```python
from build123d import *

# Parameters (mm, degrees)
F0_R          = 20
F0_R_2        = 17.5
F1_DEPTH      = 135
F2_R          = 30
F2_R_2        = 26.9985
F2_R_3        = 17.5
F3_DEPTH      = 25
F4_R          = 26.9965
F4_R_2        = 24
F4_R_3        = 17.5
F5_DEPTH      = 12
F6_R          = 25.5
F6_R_2        = 22.4965
F6_R_3        = 20
F6_R_4        = 17.5
F7_DEPTH      = 25
F8_R          = 21.9965
F8_R_2        = 17.5
F9_DEPTH      = 12
F10_S5_R      = 20
F10_T6_DEPTH  = 38
F10_S11_R     = 20
F10_T12_DEPTH = 44


# Not quite as in the source:
# - a fillet or chamfer that OpenCascade refuses, or shapes differently, is made with other operations: its cross-section is extruded or revolved along the edge and cut away or added


with BuildPart() as f1:
    # F0 (on Top) → F1 (new body)
    with BuildSketch(Plane.XY):
        Circle(F0_R)
        Circle(F0_R_2, mode=Mode.SUBTRACT)
    extrude(amount=F1_DEPTH)

    # F2 (on Top) → F3 (join)
    with BuildSketch(Plane.XY):
        Circle(F2_R)
        Circle(F2_R_2, mode=Mode.SUBTRACT)
        Circle(F2_R_2)
        Circle(F2_R_3, mode=Mode.SUBTRACT)
    extrude(amount=-F3_DEPTH)

    # F4 (on face) → F5 (cut)
    with BuildSketch(Plane(origin=(0, 0, -25), x_dir=(1, 0, 0), z_dir=(0, 0, -1))):
        Circle(F4_R)
        Circle(F4_R_2, mode=Mode.SUBTRACT)
        Circle(F4_R_2)
        Circle(F4_R_3, mode=Mode.SUBTRACT)
    extrude(amount=-F5_DEPTH, mode=Mode.SUBTRACT)

    # F6 (on face) → F7 (join)
    with BuildSketch(Plane.XY.offset(135)):
        Circle(F6_R)
        Circle(F6_R_2, mode=Mode.SUBTRACT)
        Circle(F6_R_2)
        Circle(F6_R_3, mode=Mode.SUBTRACT)
        Circle(F6_R_3)
        Circle(F6_R_4, mode=Mode.SUBTRACT)
    extrude(amount=F7_DEPTH)

    # F8 (on face) → F9 (cut)
    with BuildSketch(Plane.XY.offset(160)):
        Circle(F8_R)
        Circle(F8_R_2, mode=Mode.SUBTRACT)
    extrude(amount=-F9_DEPTH, mode=Mode.SUBTRACT)

    # F10: chamfer of 10 on 2 edges, made by hand


with BuildPart() as f10_tool2:
    # F10_s3 → F10_t4 (revolve)
    with BuildSketch(Plane.XZ):
        Polygon((15.5, 135), (25.5, 145), (25.5, 135), align=None)
    revolve(axis=Axis((0, 0, 135), (0, 0, 1)))

    # F10_s5 → F10_t6 (cut, symmetric)
    with BuildSketch(Plane.XY.offset(140)):
        Circle(F10_S5_R)
    extrude(amount=F10_T6_DEPTH, both=True, mode=Mode.SUBTRACT)


with BuildPart() as f1_1:
    add(f1.part)

    # F10_t1: cut F10_tool2
    add(f10_tool2.part, mode=Mode.SUBTRACT)


with BuildPart() as f10_tool8:
    # F10_s9 → F10_t10 (revolve)
    with BuildSketch(Plane.XZ):
        Polygon((20, 0), (30, -10), (30, 0), align=None)
    revolve(axis=Axis((0, 0, 0), (0, 0, 1)))

    # F10_s11 → F10_t12 (cut, symmetric)
    with BuildSketch(Plane.XY.offset(-5)):
        Circle(F10_S11_R)
    extrude(amount=F10_T12_DEPTH, both=True, mode=Mode.SUBTRACT)


with BuildPart() as f1_2:
    add(f1_1.part)

    # F10_t7: cut F10_tool8
    add(f10_tool8.part, mode=Mode.SUBTRACT)


solid = f1_2.part
```
The model under review builds one solid part; all positions refer to its coordinate system, in mm. A direction names the side the tool comes from. Round coordinates to 2 decimals unless told otherwise and drop trailing zeros. Order: outer loops, then holes, each group sorted by start corner. A loop starts at its lowest first (then second) coordinate and runs counter-clockwise, first axis right, second up. Notation, with made-up numbers: (-15.5, -13.75) - (-0.5, -13.75) arc R24 cw to (-0.5, 7.25) - close; hole circle Ø9 at (36.25, 37.5). An arc over 180 degrees is marked (long way). Answer in a Markdown table with one row per item.
(1) Machinability: for faces 5 (the face through (-29.97, 1.32, -17.4)), 6 (the face through (9.388, -18.049, 139.844)), 7 (the face through (-25, 11, -25)), 8 (the face through (-3.514, -26.767, -19.084)), 9 (the face through (-5.5, -24.9, 152.4)), which of the approach directions +Z, -Z, +X, -X, +Y, -Y give a long, thin tool a straight path to every point of the face, cutting with its end or side? Answer none if there is none.
Result set:
| item | result |
|---|---|
| face 5 | +Z, -Z |
| face 6 | none |
| face 7 | -Z, +X, -X, +Y, -Y |
| face 8 | -Z |
| face 9 | +Z |
(2) Mouldability with a two-part tool opening along Y and no side actions: class faces 1 (the face through (-15, -10, 148)), 2 (the face through (9.52, -18.3, -0.63)), 3 (the face through (-20.9, -7.4, 160)), 4 (the face through (0, 18, -13)) as released by +Y, released by -Y, zero draft, split by the parting line, or undercut.
Result set:
| item | result |
|---|---|
| face 1 | undercut |
| face 2 | split by the parting line |
| face 3 | zero draft |
| face 4 | undercut |
(3) Clearance check with flat-ended pins moving along their axes: P1, Ø1, axis at y = -11.5, z = 84, coming from the -X side; P2, Ø10, axis at y = -19.5, z = 21, coming from the +X side (3 decimals); P3, Ø4, axis at x = 15.5, z = 123, coming from the +Y side. State where each tip first meets the part, or that it passes through.
Result set:
| item | result |
|---|---|
| P1 | stops at x = -16.7 |
| P2 | stops at x = 13.775 |
| P3 | stops at y = 14.76 |
(4) For line 1 (Y direction, x = 0, z = -21); line 2 (Y direction, x = 0, z = 151); line 3 (X direction, y = 7.5, z = 23), list the stretches that pass through material, from the lowest coordinate up. Write a range as from..to.
Result set:
| item | result |
|---|---|
| line 1 | y = -30..-27, 27..30 |
| line 2 | y = -25.5..-22, 22..25.5 |
| line 3 | x = -18.54..-15.81, 15.81..18.54 |
(5) Take a section at A-A on x = 0. Write out the cut boundary in (y, z), plus the area to 3 significant figures.
Result set:
| item | result |
|---|---|
| outline | (-30, -25) - (-27, -25) - (-27, -13) - (-17.5, -13) - (-17.5, 148) - (-22, 148) - (-22, 160) - (-25.5, 160) - (-25.5, 145) - (-20, 139.5) - (-20, 0) - (-30, -10) - close; (17.5, -13) - (27, -13) - (27, -25) - (30, -25) - (30, -10) - (20, 0) - (20, 139.5) - (25.5, 145) - (25.5, 160) - (22, 160) - (22, 148) - (17.5, 148) - close |
| area | 1,180 mm2 |
(6) Take a section at C-C on z = 49. Write out the cut boundary in (x, y).
Result set:
| item | result |
|---|---|
| outline | circle Ø40 at (0, 0); hole circle Ø35 at (0, 0) |
